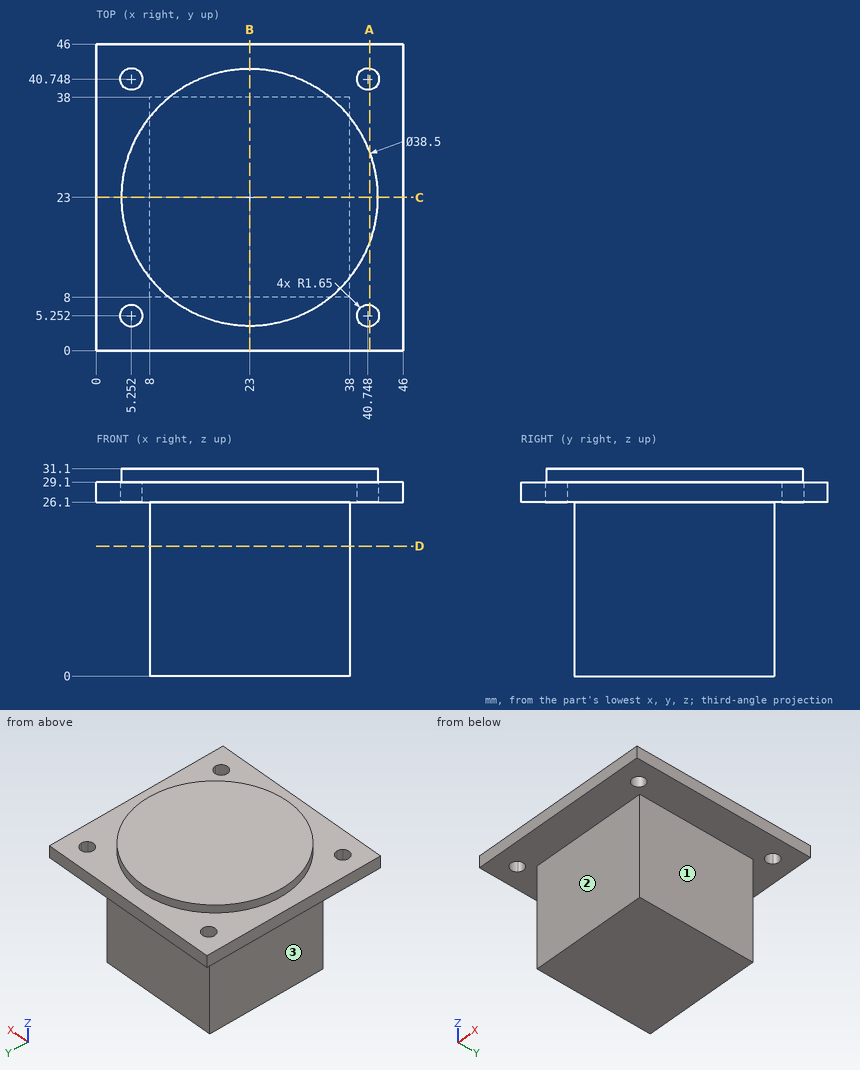
Part print with two shaded views. Sizes in mm from the minimum x, y, z corner. A direction names the side the tool comes from. Coordinates: 2 decimals unless noted, no trailing zeros. Write each loop counter-clockwise with the first axis right and the second up, starting at its lowest first coordinate (ties: lowest second). Pieces come first, ordered by that corner, then holes. Notation, with made-up numbers: (76, -25) - (115, -25) arc R13 cw to (115, -9) - close; hole circle Ø8 at (55.25, 52.25). An arc over 180 degrees is marked (long way). One line per item, written item: value. Start each with the question number.
1. Tool access for the marked faces 1, 2 and 3: list every direction of +Z, -Z, +X, -X, +Y, -Y with a clear straight run to the whole face (end or side of a thin tool).
2. Slice it at B-B (x = 23). Write the cut outline in (y, z), plus the area to 3 significant figures.
3. Slice it at A-A (x = 41). Write the cut outline in (y, z).
4. Flat gauge pins, fed straight in: pin 1 (4 mm diameter, centred on y = 24.5, z = 16, fed in from +X); pin 2 (5 mm diameter, centred on y = 19.5, z = 19.5, fed in from -X); pin 3 (13 mm diameter, centred on x = 23, z = 13.5, fed in from +Y). Where does each tip first touch, or does it go through?
5. Probe line 1 (Y direction, x = 40, z = 26.5); line 2 (Y direction, x = 32, z = 4). List the from-to ranges inside material, lowest first. Write a range as from..to.
6. Slice it at D-D (z = 19.5). Write the cut outline in (x, y), plus the area to 3 significant figures.
Answers below:
1. face 1: -Z, +X, +Y, -Y
1. face 2: -Z, +X, -X, -Y
1. face 3: -Z, -X, +Y, -Y
2. outline: (0, 26.1) - (8, 26.1) - (8, 0) - (38, 0) - (38, 26.1) - (46, 26.1) - (46, 29.1) - (42.25, 29.1) - (42.25, 31.1) - (3.75, 31.1) - (3.75, 29.1) - (0, 29.1) - close
2. area: 998 mm^2
3. outline: (0, 26.1) - (3.62, 26.1) - (3.62, 29.1) - (0, 29.1) - close; (6.88, 26.1) - (39.12, 26.1) - (39.12, 29.1) - (29.82, 29.1) - (29.82, 31.1) - (16.18, 31.1) - (16.18, 29.1) - (6.88, 29.1) - close; (42.38, 26.1) - (46, 26.1) - (46, 29.1) - (42.38, 29.1) - close
4. pin 1: stops at x = 38
4. pin 2: stops at x = 8
4. pin 3: stops at y = 38
5. line 1: y = 0..3.78, 6.72..39.28, 42.22..46
5. line 2: y = 8..38
6. outline: (8, 8) - (38, 8) - (38, 38) - (8, 38) - close
6. area: 900 mm^2
